Read the model definition and answer for the solid it produces. Units are mm, in the model's axes. Give positions to 0.01 mm unless a question says otherwise; leave off trailing zeros. Order: outer loops, then holes, each group sorted by start corner. A loop starts at its lowest first (then second) coordinate and runs counter-clockwise, first axis right, second up. Notation, with made-up numbers: (49.25, 30.25) -> (53.25, 30.25) arc R37 cw to (53.25, 67.25) -> close; hole circle Ø8 at (73.25, 59.5). An arc over 180 degrees is marked (long way). Answer as CSV lines item,"result". Start each with the question number.
1) The mould has two halves that part along X. Classify faces 1 (the face through (60, -3, 0)), 2 (the face through (-56.71, 2.797, 1.479)), 3 (the face through (153.058, -22.996, 1.479)), 4 (the face through (158.947, 2.859, 1.479)): +X half, -X half, draft (parallel to the pull), parting line (faces both ways), or undercut.
2) Find section B-B (x = 143). Determine the outline of the cut face in (y, z).
3) Find section A-A (z = 1.7). Determine the outline of the cut face in (x, y).
4) Straight lines are drawn through the part: L1, parallel to Y at x = 111, z = 0.8; L2, parallel to X at y = -4.5, z = 2.05; L3, parallel to X at y = 1, z = 2. For each, find the intervals that lie inside material, in ascending order. Write a range as from..to.
5) Flat-ended cylindrical pins translate along their axes: pin 1 Ø5 at (x, y) = (14.5, -4) entering from -Z; pin 2 Ø2.5 at (x, y) = (-53.85, -16) entering from -Z; pin 3 Ø0.9 at (x, z) = (59.5, 1.5) entering from -Y. Find the tip coordinate at first contact, or state that the pin passes through.
```python
from build123d import *

# Parameters (mm, degrees)
SKETCH_1_R      = 1.6
EXTRUDE_1_DEPTH = 3


with BuildPart() as part:
    # 草图1 → 凸台-拉伸1 (new body)
    with BuildSketch(Plane.XY):
        with BuildLine():
            Line((-53.850242828, 4), (156.149757172, 4))
            ThreePointArc((156.149757172, 4), (158.978184297, 2.828427125), (160.149757172, 0))
            Line((160.149757172, 0), (160.149757172, -16))
            ThreePointArc((160.149757172, -16), (152.900492864, -22.992597394), (146.173644012, -15.496081147))
            Line((146.173644012, -15.496081147), (146.173644012, -4))
            Line((146.173644012, -4), (-49.850242828, -4))
            Line((-49.850242828, -4), (-49.850242828, -16))
            ThreePointArc((-49.850242828, -16), (-53.850242828, -20), (-57.850242828, -16))
            Line((-57.850242828, -16), (-57.850242828, 0))
            ThreePointArc((-57.850242828, 0), (-56.678669953, 2.828427125), (-53.850242828, 4))
        make_face()
        with Locations((-53.850242828, -16)):
            Circle(SKETCH_1_R, mode=Mode.SUBTRACT)
        with BuildLine():
            Line((-49.850242828, 1.483471582), (146.173644012, 1.483471582))
            ThreePointArc((146.173644012, 1.483471582), (147.657115594, 0), (146.173644012, -1.483471582))
            Line((146.173644012, -1.483471582), (-49.850242828, -1.483471582))
            ThreePointArc((-49.850242828, -1.483471582), (-51.33371441, 0), (-49.850242828, 1.483471582))
        make_face(mode=Mode.SUBTRACT)
        with BuildLine():
            Line((149.900261056, -14.4), (156.40497097, -14.4))
            ThreePointArc((156.40497097, -14.4), (158.00497097, -16), (156.40497097, -17.6))
            Line((156.40497097, -17.6), (149.900261056, -17.6))
            ThreePointArc((149.900261056, -17.6), (148.300261056, -16), (149.900261056, -14.4))
        make_face(mode=Mode.SUBTRACT)
    extrude(amount=EXTRUDE_1_DEPTH)


solid = part.part
```
Findings below:
1,face 1,"draft"
1,face 2,"-X half"
1,face 3,"undercut"
1,face 4,"+X half"
2,outline,"(-4, 0) -> (-1.48, 0) -> (-1.48, 3) -> (-4, 3) -> close; (1.48, 0) -> (4, 0) -> (4, 3) -> (1.48, 3) -> close"
3,outline,"(-57.85, -16) arc R4 ccw to (-49.85, -16) -> (-49.85, -4) -> (146.17, -4) -> (146.17, -15.5) arc R7 ccw (long way) to (160.15, -16) -> (160.15, 0) arc R4 ccw to (156.15, 4) -> (-53.85, 4) arc R4 ccw to (-57.85, 0) -> close; hole circle Ø3.2 at (-53.85, -16); hole (-49.85, -1.48) -> (146.17, -1.48) arc R1.48 ccw to (146.17, 1.48) -> (-49.85, 1.48) arc R1.48 ccw to start; hole (149.9, -17.6) -> (156.4, -17.6) arc R1.6 ccw to (156.4, -14.4) -> (149.9, -14.4) arc R1.6 ccw to start"
4,L1,"-4..-1.48, 1.48..4"
4,L2,"-57.85..-49.85, 146.17..160.15"
4,L3,"-57.72..-50.95, 147.27..160.02"
5,pin 1,"z = 0"
5,pin 2,"through"
5,pin 3,"y = -4"
